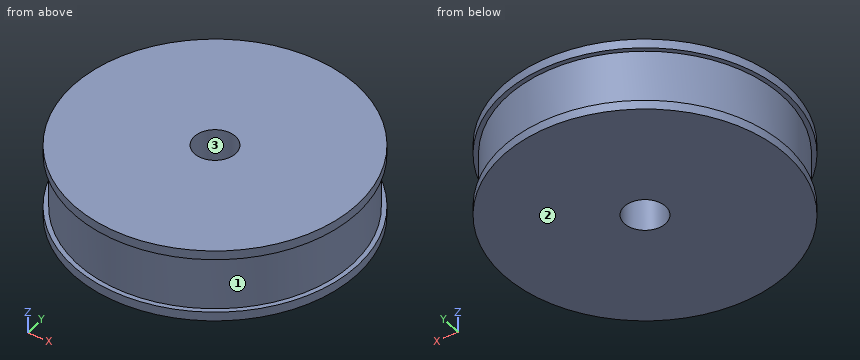
```python
from build123d import *

# Parameters (mm, degrees)
SKETCH_1_R          = 31
EXTRUDE_1_DEPTH     = 2
SKETCH_2_R          = 30
EXTRUDE_2_DEPTH     = 12
SKETCH_3_R          = 31
EXTRUDE_3_DEPTH     = 2
SKETCH_4_R          = 4.5
CUT_EXTRUDE_1_DEPTH = 47.669047558


with BuildPart() as part:
    # 草图1 → 拉伸1 (new body)
    with BuildSketch(Plane.XY):
        Circle(SKETCH_1_R)
    extrude(amount=EXTRUDE_1_DEPTH)

    # 草图2 → 拉伸2 (add)
    with BuildSketch(Plane.XY.offset(2)):
        Circle(SKETCH_2_R)
    extrude(amount=EXTRUDE_2_DEPTH)

    # 草图3 → 拉伸3 (add)
    with BuildSketch(Plane.XY.offset(14)):
        Circle(SKETCH_3_R)
    extrude(amount=EXTRUDE_3_DEPTH)

    # 草图4 → 切除-拉伸1 (cut, through all)
    with BuildSketch(Plane(origin=(0, 0, 0), x_dir=(-1, 0, 0), z_dir=(0, 0, -1))):
        Circle(SKETCH_4_R)
    extrude(amount=-CUT_EXTRUDE_1_DEPTH, mode=Mode.SUBTRACT)


solid = part.part
```
Read the model definition and answer for the solid it produces. Units are mm, in the model's axes. Face numbers are marked on the shaded views. Give positions to 0.01 mm unless a question says otherwise; leave off trailing zeros. Write each loop counter-clockwise with the first axis right and the second up, starting at its lowest first coordinate (ties: lowest second). Pieces come first, ordered by that corner, then holes. Notation, with made-up numbers: (18, -17.75) -> (30, -17.75) arc R23 ccw to (30, 8.25) -> close; hole circle Ø8 at (31, -10.5). An arc over 180 degrees is marked (long way). Answer in a Markdown table with one row per item.
1) Section A-A on y = 0 is taken. Give the vertices of the cut face in (x, z), plus the area to 3 significant figures.
Results list:
| item | result |
|---|---|
| outline | (-31, 0) -> (-4.5, 0) -> (-4.5, 16) -> (-31, 16) -> (-31, 14) -> (-30, 14) -> (-30, 2) -> (-31, 2) -> close; (4.5, 0) -> (31, 0) -> (31, 2) -> (30, 2) -> (30, 14) -> (31, 14) -> (31, 16) -> (4.5, 16) -> close |
| area | 824 mm^2 |
2) Each of these flat-tipped pins is pushed along its axis until it touches: pin 1 Ø3 at (x, z) = (-9.5, 13) entering from +Y; pin 2 Ø1 at (x, z) = (11, 4) entering from +Y; pin 3 Ø1 at (x, z) = (-19, 11) entering from +Y. Where does it stop, or does it pass through?
Results list:
| item | result |
|---|---|
| pin 1 | y = 29.85 |
| pin 2 | y = 28.1 |
| pin 3 | y = 23.62 |
3) Straight lines are drawn through the part: line 1 (Y direction, x = 0, z = 12.5); line 2 (X direction, y = -3, z = 1.25); line 3 (X direction, y = 2, z = 12.75). For each, find the intervals that lie inside material, in ascending order. Write a range as [from, to].
Results list:
| item | result |
|---|---|
| line 1 | [-30, -4.5], [4.5, 30] |
| line 2 | [-30.85, -3.35], [3.35, 30.85] |
| line 3 | [-29.93, -4.03], [4.03, 29.93] |
4) Determine the mould class of the marked faces 1, 2 and 3 for opening direction Y: released by +Y, released by -Y, zero draft, split by the parting line, or undercut.
Results list:
| item | result |
|---|---|
| face 1 | split by the parting line |
| face 2 | zero draft |
| face 3 | undercut |
5) Section D-D on y = -17 is taken. Give the vertices of the cut face in (x, z).
Results list:
| item | result |
|---|---|
| outline | (-25.92, 0) -> (25.92, 0) -> (25.92, 2) -> (24.72, 2) -> (24.72, 14) -> (25.92, 14) -> (25.92, 16) -> (-25.92, 16) -> (-25.92, 14) -> (-24.72, 14) -> (-24.72, 2) -> (-25.92, 2) -> close |
6) Section C-C on z = 7.75 is taken. Give the vertices of the cut face in (x, y), plus the area to 3 significant figures.
Results list:
| item | result |
|---|---|
| outline | circle Ø60 at (0, 0); hole circle Ø9 at (0, 0) |
| area | 2,760 mm^2 |
